Work out the finished part from the listing and answer in its coordinate system (mm). A direction names the side the tool comes from. Round coordinates to 2 decimals unless told otherwise and drop trailing zeros. Order: outer loops, then holes, each group sorted by start corner. A loop starts at its lowest first (then second) coordinate and runs counter-clockwise, first axis right, second up. Notation, with made-up numbers: M -22,0.25 L -8,0.25 A25 ccw -8,22.25 Z; hole C 26.25,-15.5 d11. An arc over 180 degrees is marked long. Answer as a JSON object with one key per item and string values. Group by question number.
from build123d import *

# Parameters (mm, degrees)
SKETCH_1_W               = 100
SKETCH_1_H               = 50
SKETCH_1_R               = 4
EXTRUDE_1_DEPTH          = 12
FILLET_1_R               = 10
FILLET_2_R               = 10
SKETCH_2_R               = 15
EXTRUDE_2_DEPTH          = 33
SKETCH_3_R               = 7.5
CUT_EXTRUDE_1_DEPTH      = 72.763500472
CUT_EXTRUDE_START        = -10
SKETCH_4_W               = 8
SKETCH_4_H               = 45
CUT_EXTRUDE_2_DEPTH      = 5
CUT_EXTRUDE_3_DEPTH      = 79.262379212
CUT_EXTRUDE_3_DEPTH_BACK = 79.262379212
SKETCH_5_R               = 4
EXTRUDE_3_DEPTH          = 8


with BuildPart() as part:
    # 草图1 → 凸台-拉伸1 (new body)
    with BuildSketch(Plane(origin=(0, 0, 0), x_dir=(1, 0, 0), z_dir=(0, 1, 0))):
        Rectangle(SKETCH_1_W, SKETCH_1_H)
        with Locations(Location((-40, 15, 0), (0, 0, 270))):
            Circle(SKETCH_1_R, mode=Mode.SUBTRACT)
        with Locations(Location((-40, -15, 0), (0, 0, 90))):
            Circle(SKETCH_1_R, mode=Mode.SUBTRACT)
        with Locations(Location((40, -15, 0), (0, 0, 270))):
            Circle(SKETCH_1_R, mode=Mode.SUBTRACT)
        with Locations(Location((40, 15, 0), (0, 0, 90))):
            Circle(SKETCH_1_R, mode=Mode.SUBTRACT)
    extrude(amount=EXTRUDE_1_DEPTH)

    # 圆角1
    fillet_1_edges = [part.edges().sort_by_distance(p)[0] for p in [
        (50, 6, -25),
    ]]
    fillet(fillet_1_edges, radius=FILLET_1_R)

    # 圆角2
    fillet_2_edges = [part.edges().sort_by_distance(p)[0] for p in [
        (-50, 6, -25),
        (50, 6, 25),
        (-50, 6, 25),
    ]]
    fillet(fillet_2_edges, radius=FILLET_2_R)

    # 草图2 → 凸台-拉伸2 (add)
    with BuildSketch(Plane(origin=(0, 12, 0), x_dir=(1, 0, 0), z_dir=(0, 1, 0))):
        with Locations(Location((0, 0, 0), (0, 0, 270))):
            Circle(SKETCH_2_R)
    extrude(amount=EXTRUDE_2_DEPTH)

    # 草图3 → 切除-拉伸1 (cut, through all)
    with BuildSketch(Plane(origin=(0, 45, 0), x_dir=(1, 0, 0), z_dir=(0, 1, 0))):
        with Locations(Location((0, 0, 0), (0, 0, 270))):
            Circle(SKETCH_3_R)
    extrude(amount=-CUT_EXTRUDE_1_DEPTH, mode=Mode.SUBTRACT)

    # 草图4 → 切除-拉伸2 (cut)
    with BuildSketch(Plane(origin=(0, 55, 0), x_dir=(1, 0, 0), z_dir=(0, 1, 0)).offset(CUT_EXTRUDE_START)):
        Rectangle(SKETCH_4_W, SKETCH_4_H)
    extrude(amount=-CUT_EXTRUDE_2_DEPTH, mode=Mode.SUBTRACT)

    # 草图5 → 切除-拉伸3 (cut, two sides: drawn at the far end of the back side and taken through both)
    with BuildSketch(Plane.XY.offset(15).offset(-CUT_EXTRUDE_3_DEPTH_BACK)):
        with Locations((0, 22)):
            Circle(SKETCH_5_R)
    extrude(amount=CUT_EXTRUDE_3_DEPTH + CUT_EXTRUDE_3_DEPTH_BACK, mode=Mode.SUBTRACT)

    # 草图8 → 凸台-拉伸3 (add)
    with BuildSketch(Plane.XY.offset(4)):
        Polygon((-50, 12), (-14.456832295, 12), (-14.456832295, 32), align=None)
    extrude_3 = extrude(amount=-EXTRUDE_3_DEPTH)

    # 镜向1: 凸台-拉伸3 across plane
    add(extrude_3.mirror(Plane(origin=(0, 0, 0), x_dir=(0, 0, 1), z_dir=(1, 0, 0))))


solid = part.part
Item 1: A tool of negligible diameter and unlimited length cuts with its end or side. For faces 5 (the flat face through (-1, 12, 17)), 6 (the flat face through (-1, 12, -17)), 7 (the flat face through (25, 18, 4)), 8 (the cylindrical face through (4.506, 28.269, 14.307)), 9 (the flat face through (4, 43, -10)), from which of +Z, -Z, +X, -X, +Y, -Y can it reach the whole face along a straight path? Write none if from no direction.
Item 2: Find section A-A (y = 22). Give the vertices of the cut face in (x, z), and give its area (3 significant figures).
Item 3: Find section B-B (z = -13). Give the vertices of the cut face in (x, y).
Item 4: Find section D-D (y = 9). Give the vertices of the cut face in (x, z), and give its area (3 significant figures).
Item 5: Each of these flat-tipped pins is pushed along its axis until it touches: pin 1 (13 mm diameter, centred on x = -40, z = -15, fed in from -Y); pin 2 (1 mm diameter, centred on y = 25.5, z = 7.5, fed in from +X); pin 3 (5 mm diameter, centred on x = 40, z = 15, fed in from -Y); pin 4 (16 mm diameter, centred on x = 37, y = 20.5, fed in from +Z). Where does it stop, or does it pass through?
Item 6: Consider L1, parallel to X at y = 3.5, z = -15; L2, parallel to X at y = 22, z = -13; L3, parallel to Y at x = 0, z = -8.5. Determine where each line is inside the solid, lowest interval first.
Item 7: The mould has two halves that part along Z. Classify faces 1 (the cylindrical face through (-43.966, 5.916, 15.521)), 2 (the flat face through (25, 18, -4)), 3 (the flat face through (10, 45, 0)), 4 (the cylindrical face through (-4.564, 22.815, -5.952)): +Z half, -Z half, draft (parallel to the pull), parting line (faces both ways), or undercut.
Item 8: Find section C-C (x = 37.5). Give the vertices of the cut face in (y, z).
Responses:
{
 "1": {"face 5": "+Z, +Y", "face 6": "-Z, +Y", "face 7": "+Z, +X, +Y", "face 8": "+Y", "face 9": "+Z, -Z, +Y"},
 "2": {"outline": "M -32.23,-4 L -14.46,-4 A15 ccw -4,-14.46 L -4,-6.34 A7.5 cw -4,6.34 L -4,14.46 A15 ccw -14.46,4 L -32.23,4 Z; M 4,-14.46 A15 ccw 14.46,-4 L 32.23,-4 L 32.23,4 L 14.46,4 A15 ccw 4,14.46 L 4,6.34 A7.5 cw 4,-6.34 Z", "area": "686 mm^2"},
 "3": {"outline": "M -50,0 L -43.46,0 L -43.46,12 L -50,12 Z; M -36.54,0 L 36.54,0 L 36.54,12 L 7.48,12 L 7.48,45 L 4,45 L 4,40 L -4,40 L -4,45 L -7.48,45 L -7.48,12 L -36.54,12 Z; M 43.46,0 L 50,0 L 50,12 L 43.46,12 Z; hole C 0,22 d8"},
 "4": {"outline": "M -50,-15 A10 ccw -40,-25 L 40,-25 A10 ccw 50,-15 L 50,15 A10 ccw 40,25 L -40,25 A10 ccw -50,15 Z; hole C -40,-15 d8; hole C -40,15 d8; hole C 0,0 d15; hole C 40,-15 d8; hole C 40,15 d8", "area": "4,540 mm^2"},
 "5": {"pin 1": "stops at y = 0", "pin 2": "stops at x = 13.27", "pin 3": "passes through", "pin 4": "stops at z = 4"},
 "6": {"L1": "x = -50 to -44, -36 to 36, 44 to 50", "L2": "x = -7.48 to -4, 4 to 7.48", "L3": "y = 0 to 18, 26 to 40"},
 "7": {"face 1": "undercut", "face 2": "-Z half", "face 3": "draft", "face 4": "undercut"},
 "8": {"outline": "M 0,-25 L 12,-25 L 12,-18.12 L 0,-18.12 Z; M 0,-11.88 L 12,-11.88 L 12,-4 L 19.03,-4 L 19.03,4 L 12,4 L 12,11.88 L 0,11.88 Z; M 0,18.12 L 12,18.12 L 12,25 L 0,25 Z"}
}
